Source: three-view drawing plus pictorial views. Frame: mm from the lowest corner of the part. A direction names the side the tool comes from. Coordinates: 2 decimals unless noted, no trailing zeros. Order: outer loops, then holes, each group sorted by start corner. A loop starts at its lowest first (then second) coordinate and runs counter-clockwise, first axis right, second up. Notation, with made-up numbers: M 86,56 L 131,56 A20 cw 131,65 Z; hole C 60,15.25 d8. An arc over 180 degrees is marked long. Use CSV: the item, a comma, the result in double quotes. Start each with the question number.
Q1. Ray query, probe 1 along Y at (x, z) = (10, 29); probe 2 along Z at (x, y) = (16.5, 2.5); probe 3 along Y at (x, z) = (19, 4.5). Return the intervals inside material, ascending.
Q2. First-contact query: P1, Ø2.5, axis at x = 24, y = 3.5, coming from the +Z side; P2, Ø1.5, axis at x = 15.5, y = 2.5, coming from the -Z side; P3, Ø1.5, axis at y = 3, z = 19.5, coming from the -X side. Flat tips, straight axial feed; report the tip coordinate or a pass-through.
Q3. Access query for the marked faces 1 and 2. Directions: +Z, -Z, +X, -X, +Y, -Y. A direction counts if a zero-diameter tool reaches every point of the face in a straight line with its end or side. Return the directions, or none.
Q4. Section query A-A, the plane z = 7.5. Output: boundary loops of the cut face in (x, y), and give its area (3 significant figures).
Q5. Section query B-B, the plane x = 14. Output: boundary loops of the cut face in (y, z), and give its area (3 significant figures).
Q6. Section query C-C, the plane x = 3. Output: boundary loops of the cut face in (y, z).
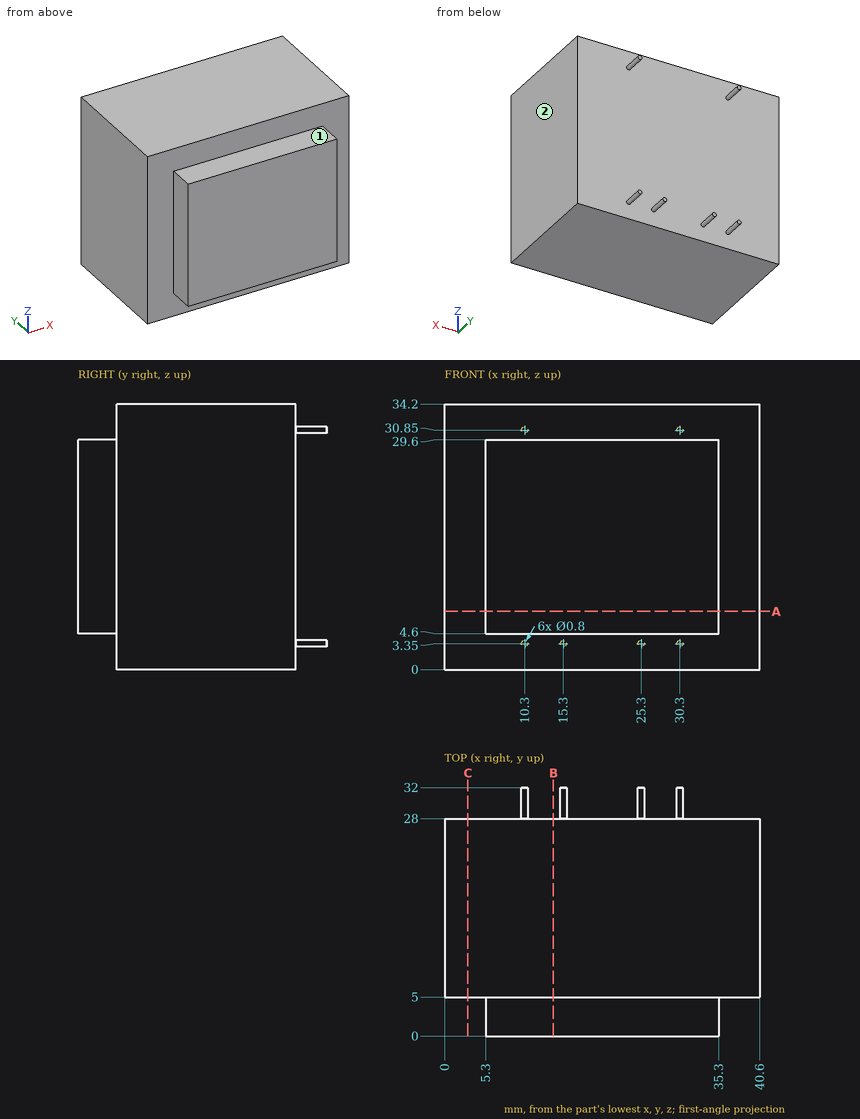
Responses:
1,probe 1,"y = 0 to 28"
1,probe 2,"z = 4.6 to 29.6"
1,probe 3,"y = 5 to 28"
2,P1,"stops at z = 29.6"
2,P2,"stops at z = 4.6"
2,P3,"stops at x = 5.3"
3,face 1,"+Z, +X, -X, -Y"
3,face 2,"+Z, -Z, +X, +Y, -Y"
4,outline,"M 0,5 L 5.3,5 L 5.3,0 L 35.3,0 L 35.3,5 L 40.6,5 L 40.6,28 L 0,28 Z"
4,area,"1,080 mm²"
5,outline,"M 0,4.6 L 5,4.6 L 5,0 L 28,0 L 28,34.2 L 5,34.2 L 5,29.6 L 0,29.6 Z"
5,area,"912 mm²"
6,outline,"M 5,0 L 28,0 L 28,34.2 L 5,34.2 Z"
